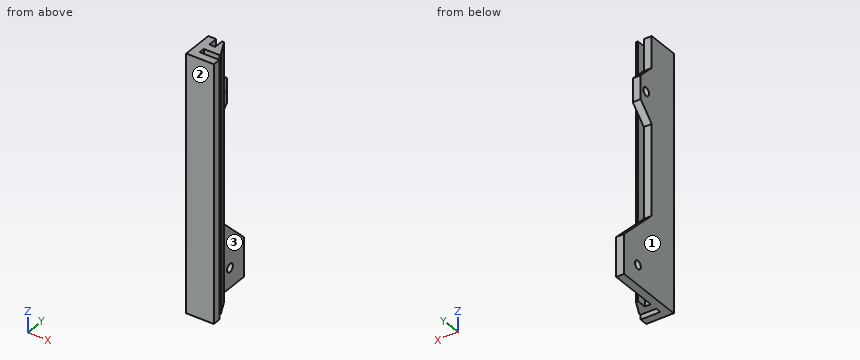
from build123d import *

# Parameters (mm, degrees)
DODANIE_WYCI_GNI_CIE1_DEPTH = 130
SZKIC2_R                    = 2.1
SZKIC2_W                    = 12
SZKIC2_H                    = 8
DODANIE_WYCI_GNI_CIE2_DEPTH = 4
SFAZOWANIE1_SIZE            = 8


with BuildPart() as part:
    # Szkic1 → Dodanie-wyciągnięcie1 (new body)
    with BuildSketch(Plane.XY):
        Polygon((0, 0), (14, 0), (14, 4), (4, 4), (4, 7), (12, 7), (12, 8), (8, 16), (7, 16), (7, 11), (4, 11), (4, 16), (0, 16), align=None)
    extrude(amount=DODANIE_WYCI_GNI_CIE1_DEPTH)

    # Szkic2 → Dodanie-wyciągnięcie2 (add)
    # profile 1 of 2: a face of its own
    with BuildSketch(Plane.ZY):
        Polygon((20, 36), (40, 16), (20, 16), (0, 16), (0, 36), align=None)
        with Locations((10, 26)):
            Circle(SZKIC2_R, mode=Mode.SUBTRACT)
    # profile 2 of 2: a face of its own
    with BuildSketch(Plane.ZY):
        with Locations((100, 20)):
            Rectangle(SZKIC2_W, SZKIC2_H)
        with Locations((100, 20)):
            Circle(SZKIC2_R, mode=Mode.SUBTRACT)
    extrude(amount=-DODANIE_WYCI_GNI_CIE2_DEPTH)

    # Sfazowanie1
    sfazowanie1_edges = [part.edges().sort_by_distance(p)[0] for p in [
        (2, 16, 94),
        (2, 16, 106),
    ]]
    chamfer(sfazowanie1_edges, length=SFAZOWANIE1_SIZE - 0.0001)  # a hair under: the kernel refuses the full size


solid = part.part
Source: CAD feature listing. Evaluate the final solid. Frame: model axes, mm. Face numbers are marked on the shaded views. Round coordinates to 2 decimals unless told otherwise and drop trailing zeros. Loops run counter-clockwise (first coordinate to the right, second up) from the corner with the lowest first, then second, coordinate; pieces in that order, holes last. Notation, with made-up numbers: (-7.5, 73) -> (14.5, 73) arc R17 cw to (14.5, 79) -> close; hole circle Ø2 at (28, 76). An arc over 180 degrees is marked (long way). Answer as a JSON object with one key per item and string values. Group by question number.
Q1. Section query A-A (y = 26). Output: boundary loops of the cut face in (x, z), plus the area to 3 significant figures.
Q2. Ray query, line 1 (Y direction, x = 4.25, z = 64); line 2 (Y direction, x = 7.75, z = 35); line 3 (Z direction, x = 3, y = 18.5). Return the intervals inside material, ascending. Write a range as from..to.
Q3. Section query B-B (z = 10). Output: boundary loops of the cut face in (x, y).
Q4. Section query C-C (x = 9.5). Output: boundary loops of the cut face in (y, z), plus the area to 3 significant figures.
Q5. Section query D-D (x = 1.75). State how many separate pieces and enclosed holes the cut face has, plus the area to 3 significant figures.
Q6. Mould query, pull axis X, two halves, no side actions, for the marked faces 1, 2 and 3. Classes: pulls with the +X half, pulls with the -X half, needs draft (parallel to the pull), parting line crosses it, or undercut.
Q7. Contact query for flat-ended pins moving along their axis: P1, Ø0.8, axis at x = 7.5, z = 73, coming from the +Y side; P2, Ø1.5, axis at y = 14.5, z = 75, coming from the -X side; P3, Ø2, axis at y = 8.5, z = 69, coming from the +X side; P4, Ø1.2, axis at x = 2, z = 100, coming from the +Y side. Output: stop coordinate, or through.
Completed:
{
 "1": {"outline": "(0, 0) -> (4, 0) -> (4, 7.9) -> (0, 7.9) -> close; (0, 12.1) -> (4, 12.1) -> (4, 30) -> (0, 30) -> close", "area": "103 mm²"},
 "2": {"line 1": "0..4, 7..11", "line 2": "0..4, 7..16", "line 3": "0..37.5, 88.5..98.53, 101.47..111.5"},
 "3": {"outline": "(0, 0) -> (14, 0) -> (14, 4) -> (4, 4) -> (4, 7) -> (12, 7) -> (12, 8) -> (8, 16) -> (7, 16) -> (7, 11) -> (4, 11) -> (4, 23.9) -> (0, 23.9) -> close; (0, 28.1) -> (4, 28.1) -> (4, 36) -> (0, 36) -> close"},
 "4": {"outline": "(0, 0) -> (4, 0) -> (4, 130) -> (0, 130) -> close; (7, 0) -> (13, 0) -> (13, 130) -> (7, 130) -> close", "area": "1,300 mm²"},
 "5": {"separate pieces": "1", "enclosed holes": "2", "area": "2,810 mm²"},
 "6": {"face 1": "pulls with the -X half", "face 2": "needs draft", "face 3": "undercut"},
 "7": {"P1": "y = 16", "P2": "x = 0", "P3": "x = 12", "P4": "y = 24"}
}
